The figure shows three views and two pictorial views of one solid part (mm, origin at its lowest corner). Answer the questions. Give positions to 0.01 mm unless a question says otherwise; leave off trailing zeros. Loops run counter-clockwise (first coordinate to the right, second up) from the corner with the lowest first, then second, coordinate; pieces in that order, holes last. Notation, with made-up numbers: M -31,21.25 L -11,21.25 A16 cw -11,34.25 Z; hole C 3,-27 d3. An arc over 180 degrees is marked long. Write item = value, one per line. Start each with the question number.
1. Section C-C on y = 10.5 is taken. Determine the outline of the cut face in (x, z).
2. The mould has two halves that part along X. Classify the marked faces 1, 2, 3 and 4: released by +X, released by -X, zero draft, split by the parting line, or undercut.
3. Section D-D on x = 23 is taken. Determine the outline of the cut face in (y, z).
4. Section A-A on x = 3.5 is taken. Determine the outline of the cut face in (y, z), plus the area to 4 significant figures.
5. A flat-ended cylindrical pin translates along its axis: pin 1 Ø3 at (x, y) = (3.5, 20) entering from +Z. Find the tip coordinate at first contact, or state that the pin passes through.
6. Section B-B on z = 12.75 is taken. Determine the outline of the cut face in (x, y).
7. Consider L1, parallel to Y at x = 3.5, z = 0.75; L2, parallel to X at y = 6, z = 13.75; L3, parallel to Z at x = 20.5, y = 31.5. Determine where each line is inside the solid, lowest interval first. Write a range as [from, to].
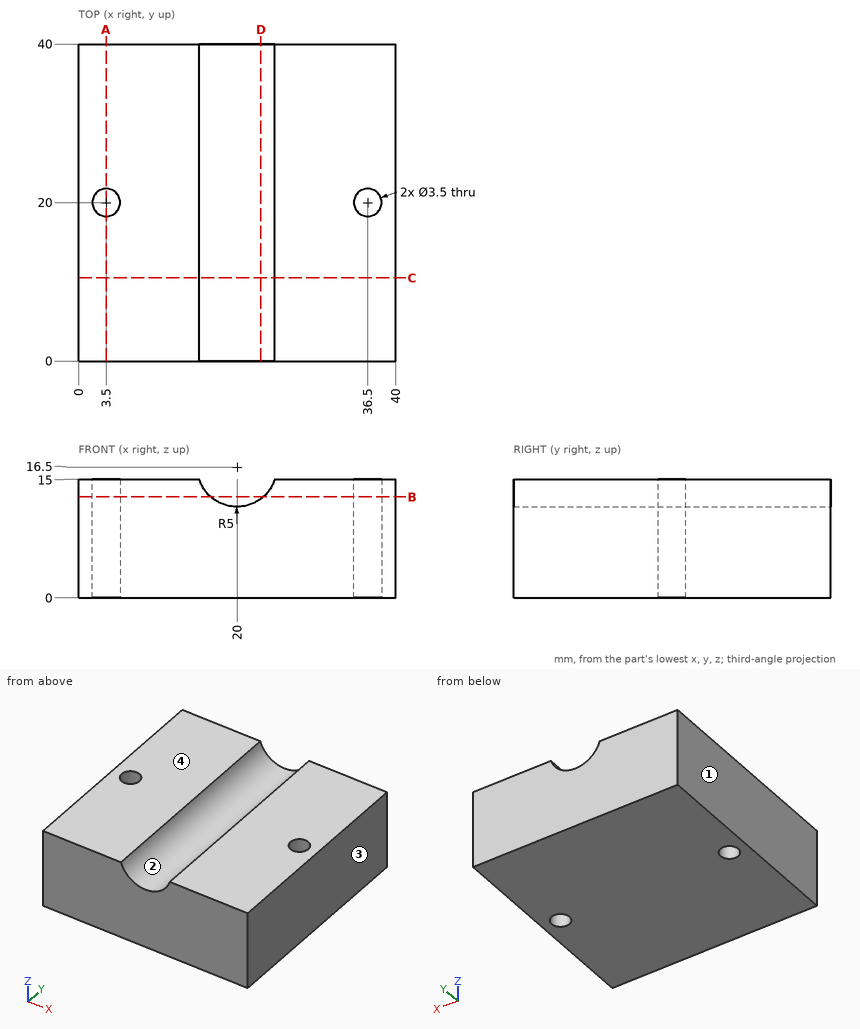
Verdict:
q1.outline = M 0,0 L 40,0 L 40,15 L 24.77,15 A5 cw 15.23,15 L 0,15 Z
q2.face_1 = released by -X
q2.face_2 = undercut
q2.face_3 = released by +X
q2.face_4 = zero draft
q3.outline = M 0,0 L 40,0 L 40,12.5 L 0,12.5 Z
q4.outline = M 0,0 L 18.25,0 L 18.25,15 L 0,15 Z; M 21.75,0 L 40,0 L 40,15 L 21.75,15 Z
q4.area = 547.5 mm2
q5.pin_1 = through
q6.outline = M 0,0 L 16.69,0 L 16.69,40 L 0,40 Z; M 23.31,0 L 40,0 L 40,40 L 23.31,40 Z; hole C 3.5,20 d3.5; hole C 36.5,20 d3.5
q7.L1 = [0, 18.25], [21.75, 40]
q7.L2 = [0, 15.82], [24.18, 40]
q7.L3 = [0, 11.53]
